Geometry: final body of the model. Coordinates: model frame, mm. A direction names the side the tool comes from. Give positions to 0.01 mm unless a question says otherwise; leave off trailing zeros. Order: outer loops, then holes, each group sorted by start corner. A loop starts at its lowest first (then second) coordinate and runs counter-clockwise, first axis right, second up. Notation, with made-up numbers: (30, 27) - (83, 27) arc R34 ccw to (83, 61) - close; hole circle Ø5 at (53.25, -36.5). An arc over 180 degrees is marked (long way). One line per item, written item: value.
Autodesk Inventor part; units mm, degrees
ref_plane "YZ Plane" through (0, 0, 0) normal (1, 0, 0) x (0, 1, 0)
ref_plane "XZ Plane" through (0, 0, 0) normal (0, 1, 0) x (-1, 0, 0)
ref_plane "XY Plane" through (0, 0, 0) normal (0, 0, 1) x (1, 0, 0)
sketch "Sketch1" plane through (0, 0, 0) normal (0, 0, 1) x (1, 0, 0)
  line L0 (-7.6738, 6.4198) -> (5.9262, 6.4198)
  line L1 (5.9262, 6.4198) -> (5.9262, -1.5802)
  line L2 (5.9262, -1.5802) -> (-7.6738, -1.5802)
  line L3 (-7.6738, -1.5802) -> (-7.6738, 6.4198)
  point P0 (0, 0)
  dimension "d0" = 8
  dimension "d1" = 13.6
extrude "Extrusion1" add sketch "Sketch1" along normal blind 21
sketch "Sketch2" plane through (5.9262, -1.5802, 0) normal (1, 0, 0) x (0, 0, -1)
  line L0 (-10.5, 7.1029) -> (-10.5, -3.9254)
  line L1 (-18.4841, 5) -> (1.1812, 5) construction
  circle A0 centre (-18, 5) radius 1.75
  circle A1 centre (-3, 5) radius 1.75
  line L2 (0, 8) -> (0, 0) construction
  line L3 (0, 8) -> (-21, 8) construction
  line L4 (-21, 0) -> (-21, 8) construction
  line L5 (0, 0) -> (-21, 0) construction
  line L6 (0, 8) -> (-21, 8) construction
  line L7 (-10.5, 8) -> (-10.5, 9.8874) construction
  point P0 (0, 1.5802)
  dimension "d4" = 3.5
  dimension "d6" = 15
  dimension "d24" = 3
extrude "Extrusion2" cut sketch "Sketch2" against normal through all
sketch "Sketch3" plane through (-7.6738, 6.4198, 0) normal (0, 1, 0) x (1, 0, 0)
  line L0 (13.6, -21) -> (0, -21)
  line L1 (6.8, -21) -> (6.8, 5.3018)
  line L2 (0, 0) -> (0, -21)
  line L3 (0, -10.5) -> (13.6, -10.5)
  line L4 (13.6, 0) -> (13.6, -21)
  circle A0 centre (6.8, -10.5) radius 3
  circle A1 centre (6.8, -10.5) radius 4.1
  point P0 (7.6738, 0)
  dimension "d9" = 6
  dimension "d10" = 8.2
extrude "bearing depth 2mm" cut sketch "Sketch3" against normal blind 4 contours A1 L3 A0 L1 | L1 A0 L3 A1 | L3 A0 L1 A1 | A1 L1 A0 L3
extrude "Extrusion4" cut sketch "Sketch3" against normal up to surface (8 mm away) contours A0 L3 L1 | L1 L3 A0 | L3 L1 A0 | L3 A0 L1
hole "Hole2" at (-0.8738, -1.5802, 10.5) direction (0, 1, 0) diameter 4 end through all counterbore diameter 8.2 counterbore depth 2.5
properties part number "slider-top-anker"
1) First-contact query: pin 1 (7 mm diameter, centred on x = -0.87, z = 10.5, fed in from -Y); pin 2 (3 mm diameter, centred on y = 3.42, z = 18, fed in from +X). Flat tips, straight axial feed; report the tip coordinate or a pass-through.
Answers below:
pin 1: y = 0.92
pin 2: through
2) Section B-B, the plane x = 0.25. Return loops of the section in (y, z), then the cut area to 3 significant figures.
Answers below:
outline: (-1.58, 0) - (6.42, 0) - (6.42, 6.56) - (2.42, 6.56) - (2.42, 7.72) - (0.92, 7.72) - (0.92, 6.56) - (-1.58, 6.56) - close; (-1.58, 14.44) - (0.92, 14.44) - (0.92, 13.28) - (2.42, 13.28) - (2.42, 14.44) - (6.42, 14.44) - (6.42, 21) - (-1.58, 21) - close; hole circle Ø3.5 at (3.42, 3); hole circle Ø3.5 at (3.42, 18)
area: 89.2 mm^2
3) Mould query, pull axis X, two halves, no side actions, for faces 1 (the face through (-0.779, 2.355, 19.389)), 2 (the face through (-7.674, 2, 10)), 3 (the face through (2, 0.92, 9)). Classes: released by +X, released by -X, zero draft, split by the parting line, or undercut.
Answers below:
face 1: zero draft
face 2: released by -X
face 3: undercut
4) Section C-C, the plane y = 5.5. Return loops of the section in (x, z).
Answers below:
outline: (-7.67, 0) - (5.93, 0) - (5.93, 21) - (-7.67, 21) - close; hole circle Ø8.2 at (-0.87, 10.5)
5) Material intervals for line 1 along X through (y, z) = (1.3, 10.5); line 2 along Z through (x, y) = (-4, 4); line 3 along Y through (x, z) = (0.5, 18), sorted ascending.
Answers below:
line 1: -7.67 to -3.87, 2.13 to 5.93
line 2: 0 to 1.35, 4.65 to 7.85, 13.15 to 16.35, 19.65 to 21
line 3: -1.58 to 1.67, 5.17 to 6.42
6) Section A-A, the plane z = 3. Return loops of the section in (x, y).
Answers below:
outline: (-7.67, -1.58) - (5.93, -1.58) - (5.93, 1.67) - (-7.67, 1.67) - close; (-7.67, 5.17) - (5.93, 5.17) - (5.93, 6.42) - (-7.67, 6.42) - close
7) Section D-D, the plane x = -3.5. Return loops of the section in (y, z).
Answers below:
outline: (-1.58, 0) - (6.42, 0) - (6.42, 7.35) - (2.42, 7.35) - (2.42, 9.05) - (0.92, 9.05) - (0.92, 7.35) - (-1.58, 7.35) - close; (-1.58, 13.65) - (0.92, 13.65) - (0.92, 11.95) - (2.42, 11.95) - (2.42, 13.65) - (6.42, 13.65) - (6.42, 21) - (-1.58, 21) - close; hole circle Ø3.5 at (3.42, 3); hole circle Ø3.5 at (3.42, 18)
8) Set-up query: faces 4 (the face through (-1.054, -0.313, 14.596)), 5 (the face through (-1, 2.42, 14)), 6 (the face through (-1.264, 1.68, 7.526)). Return all of +Z, -Z, +X, -X, +Y, -Y with unobstructed straight access to the full face (end or side cutting, diameter ignored); none if empty.
Answers below:
face 4: -Y
face 5: +Y
face 6: +Y, -Y
